The model under review builds one solid part; all positions refer to its coordinate system, in mm. Coordinates: 2 decimals unless noted, no trailing zeros. Write each loop counter-clockwise with the first axis right and the second up, starting at its lowest first coordinate (ties: lowest second). Pieces come first, ordered by that corner, then holes. Notation, with made-up numbers: (-15.75, 30) - (0.25, 30) arc R18 ccw to (0.25, 57) - close; hole circle Ø3 at (28, 72.5). An arc over 180 degrees is marked (long way). Put each result on its own line as item: value. Start each with the question number.
Item 1: Consider section B-B on z = 0. Give the boundary of the cut face in (x, y).
Item 2: To check wall thickness, follow L1, parallel to Y at x = -41.75, z = 0; L2, parallel to X at y = 25, z = -4.5. State the ranges of each line that lie inside material, in increasing order. Write a range as [from, to].
Item 3: For pin 1 (3 mm diameter, centred on y = 24.5, z = 2.5, fed in from -X) (3 decimals); pin 2 (16 mm diameter, centred on y = 25, z = 0, fed in from -X) (3 decimals), all flat-tipped, find the tip position at first contact; note any pin that passes through.
Item 4: Consider section A-A on y = 25. Give the boundary of the cut face in (x, z).
```python
from build123d import *

# Parameters (mm, degrees)
SKETCH1_W           = 99.270032964
SKETCH1_H           = 35
BOSS_EXTRUDE1_DEPTH = 50
SKETCH2_R           = 5
CUT_EXTRUDE1_DEPTH  = 10
SKETCH3_R           = 5
CUT_EXTRUDE2_DEPTH  = 10


with BuildPart() as part:
    # Sketch1 → Boss-Extrude1 (new body)
    with BuildSketch(Plane(origin=(0, 0, 0), x_dir=(1, 0, 0), z_dir=(0, 1, 0))):
        Rectangle(SKETCH1_W, SKETCH1_H)
    extrude(amount=BOSS_EXTRUDE1_DEPTH)

    # Sketch2 → Cut-Extrude1 (cut)
    with BuildSketch(Plane.ZY.offset(49.635016482)):
        with Locations((0, 25)):
            Circle(SKETCH2_R)
    extrude(amount=-CUT_EXTRUDE1_DEPTH, mode=Mode.SUBTRACT)

    # Sketch3 → Cut-Extrude2 (cut)
    with BuildSketch(Plane(origin=(49.635016482, 0, 0), x_dir=(0, 0, -1), z_dir=(1, 0, 0))):
        with Locations((0, 25)):
            Circle(SKETCH3_R)
    extrude(amount=-CUT_EXTRUDE2_DEPTH, mode=Mode.SUBTRACT)


solid = part.part
```
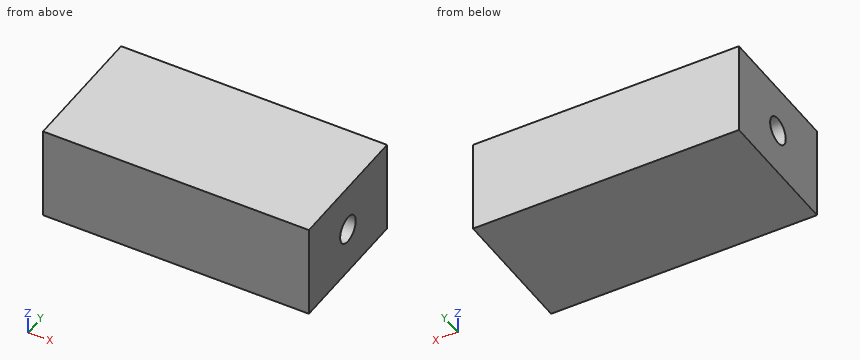
Report:
1. outline: (-49.64, 0) - (49.64, 0) - (49.64, 20) - (39.64, 20) - (39.64, 30) - (49.64, 30) - (49.64, 50) - (-49.64, 50) - (-49.64, 30) - (-39.64, 30) - (-39.64, 20) - (-49.64, 20) - close
2. L1: [0, 20], [30, 50]
2. L2: [-39.64, 39.64]
3. pin 1: x = -39.635
3. pin 2: x = -49.635
4. outline: (-49.64, -17.5) - (49.64, -17.5) - (49.64, -5) - (39.64, -5) - (39.64, 5) - (49.64, 5) - (49.64, 17.5) - (-49.64, 17.5) - (-49.64, 5) - (-39.64, 5) - (-39.64, -5) - (-49.64, -5) - close
